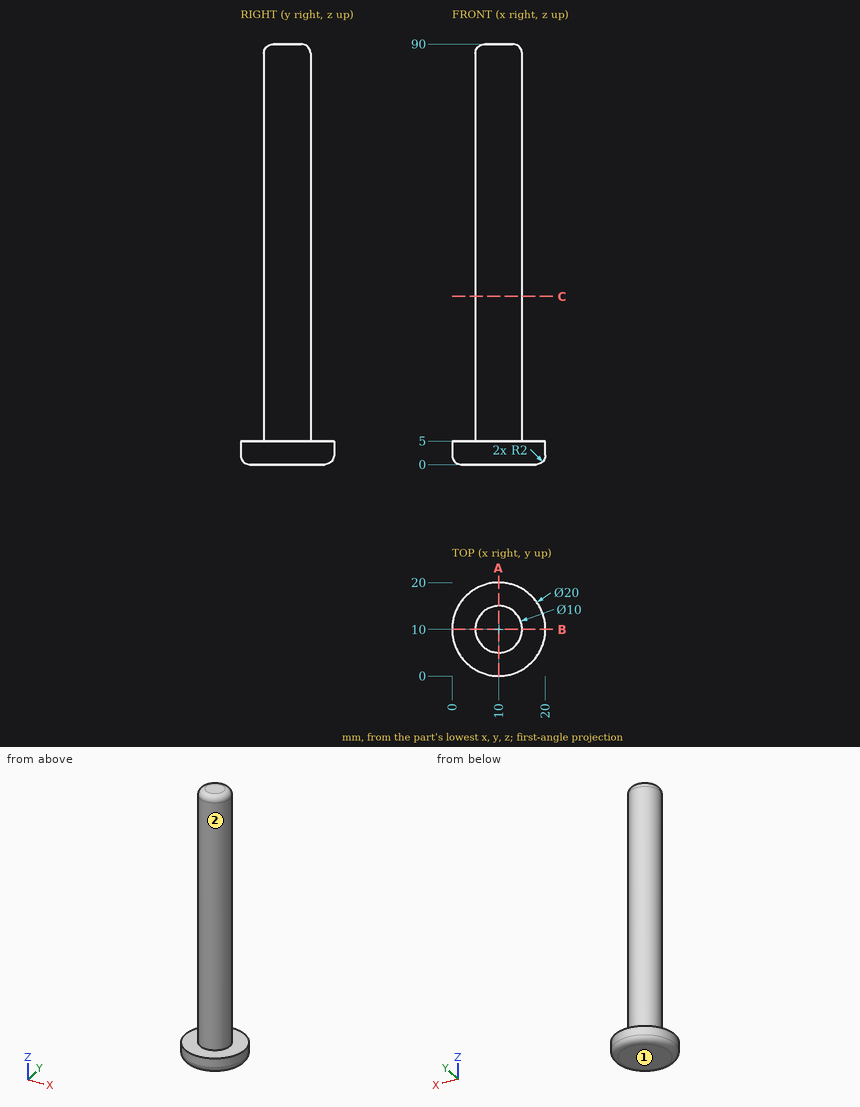
Design review of the part shown in the three views and the two pictorial views. Dimensions are in mm from the part's minimum x, y and z. A direction names the side the tool comes from. Give positions to 0.01 mm unless a question says otherwise; leave off trailing zeros. Write each loop counter-clockwise with the first axis right and the second up, starting at its lowest first coordinate (ties: lowest second). Pieces come first, ordered by that corner, then holes.
(1) Clearance check with flat-ended pins moving along their axes: pin 1 Ø12 at (y, z) = (4.5, 75) entering from -X; pin 2 Ø1.5 at (x, y) = (9, 16) entering from +Z; pin 3 Ø2 at (y, z) = (11, 16.5) entering from +X; pin 4 Ø2 at (y, z) = (17, 52.5) entering from -X. State where each tip first meets the part, or that it passes through.
Checked values:
pin 1: stops at x = 5
pin 2: stops at z = 5
pin 3: stops at x = 15
pin 4: passes through
(2) Add section A-A (x = 10). Give the boundary of the cut face in (y, z), and give its area (3 significant figures).
Checked values:
outline: (0, 2) arc R2 ccw to (2, 0) - (18, 0) arc R2 ccw to (20, 2) - (20, 5) - (15, 5) - (15, 88) arc R2 ccw to (13, 90) - (7, 90) arc R2 ccw to (5, 88) - (5, 5) - (0, 5) - close
area: 947 mm2
(3) Wall thickness on line 1 along Z through (x, y) = (7, 16.5); line 2 along Y through (x, z) = (10.25, 20); line 3 along X through (y, z) = (13, 79): over which ranges is each line inside the solid? List them lowest first.
Checked values:
line 1: z = 0 to 5
line 2: y = 5.01 to 14.99
line 3: x = 6 to 14
(4) Tool access review of the marked faces 1 and 2: name each direction out of +Z, -Z, +X, -X, +Y, -Y from which nothing blocks a thin tool from reaching the whole face with its end or side.
Checked values:
face 1: -Z, +X, -X, +Y, -Y
face 2: +Z
(5) Add section C-C (z = 36). Give the boundary of the cut face in (x, y), and give its area (3 significant figures).
Checked values:
outline: circle Ø10 at (10, 10)
area: 78.5 mm2
